Source: CAD feature listing. Evaluate the final solid. Frame: model axes, mm. Face numbers are marked on the shaded views. Give positions to 0.01 mm unless a question says otherwise; leave off trailing zeros. Loops run counter-clockwise (first coordinate to the right, second up) from the corner with the lowest first, then second, coordinate; pieces in that order, holes last. Notation, with made-up numbers: (58, -3) -> (83, -3) arc R23 ccw to (83, 17) -> close; hole circle Ø10 at (80.5, -1.75). An arc over 180 degrees is marked (long way). Return JSON: item names as keys, results as strings. Group by question number.
(1) Cut plane C-C on z = 10.5. Return loops of the section in (x, y).
(2) Ray query, line 1 (Y direction, x = -0.5, z = 9.25); line 2 (Y direction, x = 7, z = 6); line 3 (X direction, y = 35, z = 3.75). Return the intervals inside material, ascending. Write a range as from..to.
(3) Draft query along Y for the marked faces 1, 2 and 3. Return one class per face: released by +Y, released by -Y, zero draft, split by the parting line, or undercut.
(4) Cut plane A-A on x = 0. Return loops of the section in (y, z).
(5) Pin query (flat end, axial travel): pin 1 (2 mm diameter, centred on x = 17, z = 9, fed in from -Y); pin 2 (2 mm diameter, centred on x = 32.5, z = 1.5, fed in from -Y); pin 3 (3 mm diameter, centred on x = 42.97, y = 12.32, fed in from -Z); pin 4 (2 mm diameter, centred on x = -35.5, z = 2, fed in from +Y). Return the tip coordinate at first contact, or that it passes through.
```python
from build123d import *

# Parameters (mm, degrees)
F0_R     = 47.2105080962
F0_R_2   = 40.4501471724
F1_DEPTH = 25.4
F2_DEPTH = 12.7
F4_D     = 2.4


with BuildPart() as f1:
    # F0 (on Top) → F1 (new body)
    with BuildSketch(Plane.XY):
        Circle(F0_R)
        Circle(F0_R_2, mode=Mode.SUBTRACT)
    extrude(amount=F1_DEPTH)

    # F2 (cut): a face of the model
    f2_faces = [f1.faces().sort_by_distance(p)[0] for p in [
        (-45.8751932795, 0, 25.4),
    ]]
    extrude(f2_faces, amount=-F2_DEPTH, mode=Mode.SUBTRACT)

    # F4 (through all)
    with Locations(Plane.XY.offset(12.7)):
        with Locations((42.9688580334, 12.3208649457)):
            Hole(F4_D / 2)


solid = f1.part
```
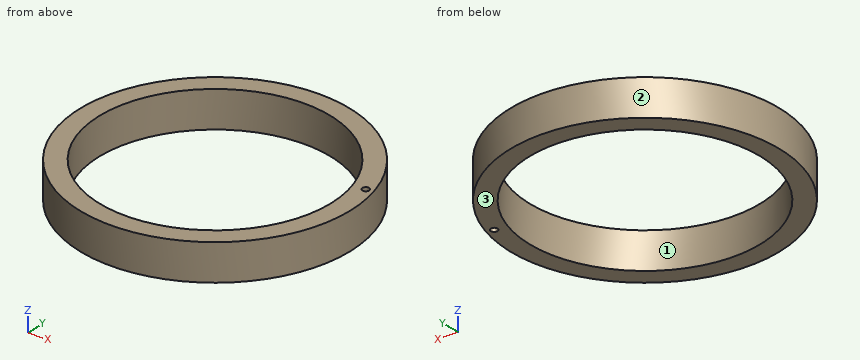
Answers:
{
 "1": {"outline": "circle Ø94.42 at (0, 0); hole circle Ø80.9 at (0, 0); hole circle Ø2.4 at (42.97, 12.32)"},
 "2": {"line 1": "-47.21..-40.45, 40.45..47.21", "line 2": "-46.69..-39.84, 39.84..46.69", "line 3": "-31.68..-20.28, 20.28..31.68"},
 "3": {"face 1": "undercut", "face 2": "split by the parting line", "face 3": "zero draft"},
 "4": {"outline": "(-47.21, 0) -> (-40.45, 0) -> (-40.45, 12.7) -> (-47.21, 12.7) -> close; (40.45, 0) -> (47.21, 0) -> (47.21, 12.7) -> (40.45, 12.7) -> close"},
 "5": {"pin 1": "y = -44.42", "pin 2": "y = -35.17", "pin 3": "z = 0", "pin 4": "y = 32.23"}
}
